from build123d import *

# Parameters (mm, degrees)
BOSS_EXTRUDE1_DEPTH = 110
BOSS_EXTRUDE2_START = -3
BOSS_EXTRUDE2_DEPTH = 3
LPATTERN1_COUNT     = 15
LPATTERN1_PITCH     = 7


with BuildPart() as part:
    # Sketch1 → Boss-Extrude1 (new body)
    with BuildSketch(Plane(origin=(0, 0, 0), x_dir=(1, 0, 0), z_dir=(0, 1, 0))):
        with BuildLine():
            Line((0, 0), (13, 0))
            ThreePointArc((13, 0), (38, 25), (63, 0))
            Line((63, 0), (78, 0))
            ThreePointArc((78, 0), (103, 25), (128, 0))
            Line((128, 0), (143, 0))
            ThreePointArc((143, 0), (168, 25), (193, 0))
            Line((193, 0), (208, 0))
            ThreePointArc((208, 0), (233, 25), (258, 0))
            Line((258, 0), (271, 0))
            Line((271, 0), (271, 55))
            ThreePointArc((271, 55), (268.071067812, 62.071067812), (261, 65))
            Line((261, 65), (10, 65))
            ThreePointArc((10, 65), (2.928932188, 62.071067812), (0, 55))
            Line((0, 55), (0, 0))
        make_face()
    extrude(amount=BOSS_EXTRUDE1_DEPTH)

    # Sketch3 → Boss-Extrude2 (add)
    with BuildSketch(Plane(origin=(0, 110, 0), x_dir=(1, 0, 0), z_dir=(0, 1, 0)).offset(BOSS_EXTRUDE2_START)):
        with BuildLine():
            Line((277, 0), (277, 55))
            ThreePointArc((277, 55), (272.313708499, 66.313708499), (261, 71))
            Line((261, 71), (10, 71))
            ThreePointArc((10, 71), (-1.313708499, 66.313708499), (-6, 55))
            Line((-6, 55), (-6, 0))
            Line((-6, 0), (0, 0))
            Line((0, 0), (0, 55))
            ThreePointArc((0, 55), (2.928932188, 62.071067812), (10, 65))
            Line((10, 65), (261, 65))
            ThreePointArc((261, 65), (268.071067812, 62.071067812), (271, 55))
            Line((271, 55), (271, 0))
            Line((271, 0), (277, 0))
        make_face()
    boss_extrude2 = extrude(amount=BOSS_EXTRUDE2_DEPTH)

    # LPattern1: Boss-Extrude2 ×15
    with Locations(*[(0, -i * LPATTERN1_PITCH, 0) for i in range(1, LPATTERN1_COUNT)]):
        add(boss_extrude2)


solid = part.part
Read the model definition and answer for the solid it produces. Units are mm, in the model's axes. A direction names the side the tool comes from. Give positions to 0.01 mm unless a question says otherwise; leave off trailing zeros. Use CSV: the item, a comma, the result in double quotes. Start each with the question number.
(1) Determine the mould class of faces 6 (the flat face through (134, 0, -40)), 7 (the cylindrical face through (3.01, 20.97, -62.15)), 8 (the cylindrical face through (272.437, 94.479, -66.189)), 9 (the cylindrical face through (3.01, 48.97, -62.15)) for opening direction Y: +Y half, -Y half, draft (parallel to the pull), parting line (faces both ways), or undercut.
(2) Given P1, Ø1.2, axis at y = 85, z = -34, coming from the -X side; P2, Ø2, axis at x = 125.5, y = 62.5, coming from the -Z side; P3, Ø1.2, axis at y = 69, z = -29, coming from the +X side, each flat-ended and moving along its own axis, determine where each tip first touches the part or whether it passes through.
(3) Consider line 1 along X through (y, z) = (55, -45.5); line 2 along Z through (x, y) = (175.5, 51.5); line 3 along Z through (x, y) = (156, 11.5). Determine where each line is inside the solid, lowest interval first.
(4) For faces 1 (the cylindrical face through (3.01, 83.97, -62.15)), 2 (the flat face through (135, 9, -67)), 3 (the cylindrical face through (272.437, 31.479, -66.189)), 4 (the flat face through (135, 65, -67)), 5 (the flat face through (137, 4, -65)), determine the directions among +Z, -Z, +X, -X, +Y, -Y from which every point of the face is accessible in a straight line to the end or side of a thin tool.
(5) Find section A-A (z = -9). Count the separate pieces of the cut face and the enclosed holes in it, plus the area to 3 significant figures.
Findings below:
1,face 6,"-Y half"
1,face 7,"undercut"
1,face 8,"draft"
1,face 9,"undercut"
2,P1,"x = 0"
2,P2,"z = -65"
2,P3,"x = 271"
3,line 1,"0 to 271"
3,line 2,"-71 to -23.85"
3,line 3,"-71 to -21.93"
4,face 1,"-Z, -X"
4,face 2,"-Z, -Y"
4,face 3,"-Z, +X, +Y, -Y"
4,face 4,"-Z"
4,face 5,"-Z, +X, -X, -Y"
5,separate pieces,"5"
5,enclosed holes,"0"
5,area,"9,830 mm2"
